Input: part model. Units: mm. Frame: model coordinates. Face numbers are marked on the shaded views. A direction names the side the tool comes from. Coordinates: 2 decimals unless noted, no trailing zeros. Write each loop counter-clockwise with the first axis right and the second up, starting at its lowest first coordinate (ties: lowest second). Pieces come first, ordered by that corner, then holes. Notation, with made-up numbers: (-29.75, 54.5) - (17.25, 54.5) arc R24 cw to (17.25, 93.5) - close; hole circle Ø8 at (-14.75, 1). An arc over 180 degrees is marked (long way). Put each result on its own line as item: value. Start each with the question number.
1. Cut plane B-B, the plane x = -24.5. Return loops of the section in (y, z), and give its area (3 significant figures).
2. Cut plane C-C, the plane z = 7. Count the separate pieces of the cut face and the enclosed holes in it, and give its area (3 significant figures).
3. Cut plane D-D, the plane x = 12. Return loops of the section in (y, z), and give its area (3 significant figures).
4. Cut plane A-A, the plane z = 24.75. Return loops of the section in (x, y), and give its area (3 significant figures).
5. Pin query (flat end, axial travel): pin 1 (8 mm diameter, centred on x = -16, y = 3.5, fed in from +Z). Return the tip coordinate at first contact, or that it passes through.
6. Access query for the marked faces 5 and 6. Directions: +Z, -Z, +X, -X, +Y, -Y. A direction counts if a zero-diameter tool reaches every point of the face in a straight line with its end or side. Return the directions, or none.
7. Line query: line 1 (Y direction, x = 0, z = 3.6); line 2 (Y direction, x = 6, z = 8.25); line 3 (Y direction, x = -5, z = 8). Output: solid intervals per line, ascending.
8. Pull-direction query (X, two-part tool) for the marked faces 1, 2, 3 and 4; classes: released by +X, released by -X, zero draft, split by the parting line, or undercut.
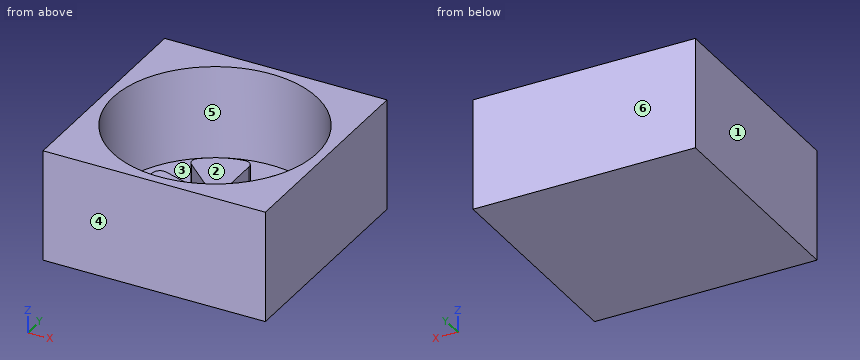
from build123d import *

# Parameters (mm, degrees)
CROQUIS1_R              = 30
SALIENTE_EXTRUIR1_DEPTH = 30
CROQUIS2_R              = 27.5
CORTAR_EXTRUIR1_DEPTH   = 25
CROQUIS3_R              = 2.5
SALIENTE_EXTRUIR2_DEPTH = 5
CROQUIS4_R              = 5.5
CROQUIS4_R_2            = 2.5
CORTAR_EXTRUIR2_DEPTH   = 2
CROQUIS6_W              = 60
CROQUIS6_H              = 60
CROQUIS6_R              = 27.5
SALIENTE_EXTRUIR3_DEPTH = 30
SALIENTE_EXTRUIR5_DEPTH = 5
REDONDEO1_R             = 2


with BuildPart() as part:
    # Croquis1 → Saliente-Extruir1 (new body)
    with BuildSketch(Plane.XY):
        Circle(CROQUIS1_R)
    extrude(amount=SALIENTE_EXTRUIR1_DEPTH)

    # Croquis2 → Cortar-Extruir1 (cut)
    with BuildSketch(Plane.XY.offset(30)):
        Circle(CROQUIS2_R)
    extrude(amount=-CORTAR_EXTRUIR1_DEPTH, mode=Mode.SUBTRACT)

    # Croquis3 → Saliente-Extruir2 (add)
    with BuildSketch(Plane.XY.offset(5)):
        Circle(CROQUIS3_R)
    extrude(amount=SALIENTE_EXTRUIR2_DEPTH)

    # Croquis4 → Cortar-Extruir2 (cut)
    with BuildSketch(Plane.XY.offset(5)):
        Circle(CROQUIS4_R)
        Circle(CROQUIS4_R_2, mode=Mode.SUBTRACT)
    extrude(amount=-CORTAR_EXTRUIR2_DEPTH, mode=Mode.SUBTRACT)

    # Croquis6 → Saliente-Extruir3 (add)
    with BuildSketch(Plane.XY.offset(30)):
        Rectangle(CROQUIS6_W, CROQUIS6_H)
        Circle(CROQUIS6_R, mode=Mode.SUBTRACT)
    extrude(amount=-SALIENTE_EXTRUIR3_DEPTH)

    # Croquis7 → Saliente-Extruir5 (add)
    with BuildSketch(Plane.XY.offset(5)):
        with BuildLine():
            Line((0, 6), (0, 19))
            ThreePointArc((0, 19), (-7.727996218, 17.357363695), (-14.119751684, 12.713481521))
            Line((-14.119751684, 12.713481521), (-4.458868953, 4.014783638))
            ThreePointArc((-4.458868953, 4.014783638), (-2.440419858, 5.481272746), (0, 6))
        make_face()
        with BuildLine():
            Line((2.440419858, 5.481272746), (7.727996218, 17.357363695))
            ThreePointArc((7.727996218, 17.357363695), (14.119751684, 12.713481521), (18.07007381, 5.871322893))
            Line((18.07007381, 5.871322893), (5.706339098, 1.854101966))
            ThreePointArc((5.706339098, 1.854101966), (4.458868953, 4.014783638), (2.440419858, 5.481272746))
        make_face()
        with BuildLine():
            Line((5.967131372, -0.62717078), (18.895916012, -1.986040802))
            ThreePointArc((18.895916012, -1.986040802), (16.454482672, -9.5), (11.167919794, -15.371322893))
            Line((11.167919794, -15.371322893), (3.526711514, -4.854101966))
            ThreePointArc((3.526711514, -4.854101966), (5.196152423, -3), (5.967131372, -0.62717078))
        make_face()
        with BuildLine():
            Line((1.247470145, -5.868885604), (3.950322126, -18.584804414))
            ThreePointArc((3.950322126, -18.584804414), (-3.950322126, -18.584804414), (-11.167919794, -15.371322893))
            Line((-11.167919794, -15.371322893), (-3.526711514, -4.854101966))
            ThreePointArc((-3.526711514, -4.854101966), (-1.247470145, -5.868885604), (1.247470145, -5.868885604))
        make_face()
        with BuildLine():
            Line((-5.196152423, -3), (-16.454482672, -9.5))
            ThreePointArc((-16.454482672, -9.5), (-18.895916012, -1.986040802), (-18.07007381, 5.871322893))
            Line((-18.07007381, 5.871322893), (-5.706339098, 1.854101966))
            ThreePointArc((-5.706339098, 1.854101966), (-5.967131372, -0.62717078), (-5.196152423, -3))
        make_face()
    extrude(amount=SALIENTE_EXTRUIR5_DEPTH)

    # Redondeo1
    redondeo1_edges = [part.edges().sort_by_distance(p)[0] for p in [
        (-4.458868953, 4.014783638, 7.5),
        (0, 6, 7.5),
        (0, 19, 7.5),
        (-14.119751684, 12.713481521, 7.5),
        (2.440419858, 5.481272746, 7.5),
        (5.706339098, 1.854101966, 7.5),
        (18.07007381, 5.871322893, 7.5),
        (7.727996218, 17.357363695, 7.5),
        (5.967131372, -0.62717078, 7.5),
        (3.526711514, -4.854101966, 7.5),
        (11.167919794, -15.371322893, 7.5),
        (18.895916012, -1.986040802, 7.5),
        (1.247470145, -5.868885604, 7.5),
        (-3.526711514, -4.854101966, 7.5),
        (-11.167919794, -15.371322893, 7.5),
        (3.950322126, -18.584804414, 7.5),
        (-5.196152423, -3, 7.5),
        (-5.706339098, 1.854101966, 7.5),
        (-18.07007381, 5.871322893, 7.5),
        (-16.454482672, -9.5, 7.5),
    ]]
    fillet(redondeo1_edges, radius=REDONDEO1_R)


solid = part.part
Report:
1. outline: (-30, 0) - (30, 0) - (30, 30) - (12.49, 30) - (12.49, 5) - (-12.49, 5) - (-12.49, 30) - (-30, 30) - close
1. area: 1,180 mm^2
2. separate pieces: 7
2. enclosed holes: 1
2. area: 1,910 mm^2
3. outline: (-30, 0) - (30, 0) - (30, 30) - (24.74, 30) - (24.74, 5) - (14.73, 5) - (14.73, 10) - (3.9, 10) - (3.9, 5) - (-1.26, 5) - (-1.26, 10) - (-14.43, 10) - (-14.43, 5) - (-24.74, 5) - (-24.74, 30) - (-30, 30) - close
3. area: 683 mm^2
4. outline: (-30, -30) - (30, -30) - (30, 30) - (-30, 30) - close; hole circle Ø55 at (0, 0)
4. area: 1,220 mm^2
5. pin 1: stops at z = 10
6. face 5: +Z
6. face 6: +Z, -Z, +X, -X, +Y
7. line 1: y = -30 to -5.5, -2.5 to 2.5, 5.5 to 30
7. line 2: y = -30 to -26.84, -8.26 to -1.47, 2.44 to 13.48, 26.84 to 30
7. line 3: y = -30 to -27.04, -18.33 to -6.88, 4.76 to 18.33, 27.04 to 30
8. face 1: released by -X
8. face 2: undercut
8. face 3: undercut
8. face 4: zero draft
